```python
from build123d import *

# Parameters (mm, degrees)
F0_W      = 45.72
F0_H      = 7.62
F1_DEPTH  = 25.4
F2_DEPTH  = 25.4
F3_DEPTH  = 3.81
F4_R      = 5.08
F7_DEPTH  = 3.81
F10_DEPTH = 3.81
F11_R     = 1.27


with BuildPart() as f1:
    # F0 (on Front) → F1 (new body, symmetric)
    with BuildSketch(Plane.XZ):
        with Locations((-3.917041, 3.81)):
            Rectangle(F0_W, F0_H)
    extrude(amount=F1_DEPTH, both=True)

    # F0 (on Front) → F2 (join, symmetric)
    with BuildSketch(Plane.XZ):
        Polygon((26.562959, 38.1), (18.942959, 38.1), (18.942959, 7.62), (18.942959, 0), (18.942959, -7.62), (26.562959, -7.62), align=None)
    extrude(amount=F2_DEPTH, both=True)

    # F0 (on Front) → F3 (join, symmetric)
    with BuildSketch(Plane.XZ):
        with BuildLine():
            Line((18.942959, -7.62), (18.942959, 0))
            Line((18.942959, 0), (-26.777041, 0))
            add(Edge.make_bspline(
                [(-26.777041, 0), (-8.442144, -4.630308), (0.605608, -7.060291), (18.942959, -7.62)],
                knots=[0, 0, 0, 0, 46.35065, 46.35065, 46.35065, 46.35065], degree=3))
        make_face()
    extrude(amount=F3_DEPTH, both=True)

    # F4
    f4_edges = [f1.edges().sort_by_distance(p)[0] for p in [
        (22.752959, -25.4, -7.62),
        (22.752959, 25.4, -7.62),
        (22.752959, 25.4, 38.1),
        (22.752959, -25.4, 38.1),
        (-26.777041, 25.4, 3.81),
        (-26.777041, -25.4, 3.81),
    ]]
    fillet(f4_edges, radius=F4_R)

    # F6 (on offset) → F7 (join, symmetric)
    with BuildSketch(Plane.XZ.offset(12.7)):
        with BuildLine():
            Line((19.504473, 7.642324), (19.504473, 37.258741))
            add(Edge.make_bspline(
                [(19.504473, 37.258741), (-2.269479, 32.051925), (-15.974103, 23.058929), (-26.861079, 7.675159)],
                knots=[0, 0, 0, 0, 54.99957, 54.99957, 54.99957, 54.99957], degree=3))
            Line((-26.861079, 7.675159), (19.504473, 7.642324))
        make_face()
    extrude(amount=F7_DEPTH, both=True)

    # F9 (on offset) → F10 (join, symmetric)
    with BuildSketch(Plane.XZ.offset(-12.7)):
        with BuildLine():
            Line((19.418189, 7.557305), (19.418189, 37.171504))
            add(Edge.make_bspline(
                [(19.418189, 37.171504), (-2.355763, 31.964688), (-16.060385, 22.97391), (-26.947361, 7.590141)],
                knots=[0, 0, 0, 0, 54.998375, 54.998375, 54.998375, 54.998375], degree=3))
            Line((-26.947361, 7.590141), (19.418189, 7.557305))
        make_face()
    extrude(amount=F10_DEPTH, both=True)

    # F11
    f11_edges = [f1.edges().sort_by_distance(p)[0] for p in [
        (26.562959, 25.4, 15.24),
        (26.562959, 23.912102, -6.132102),
        (26.562959, 23.912102, 36.612102),
        (26.562959, 0, -7.62),
        (26.562959, 0, 38.1),
        (26.562959, -23.912102, -6.132102),
        (26.562959, -23.912102, 36.612102),
        (26.562959, -25.4, 15.24),
        (-6.865306, -16.51, 26.848425),
        (-6.865306, -8.89, 26.848425),
        (-6.913699, 16.51, 26.785701),
        (-6.913699, 8.89, 26.785701),
    ]]
    fillet(f11_edges, radius=F11_R)


solid = f1.part
```
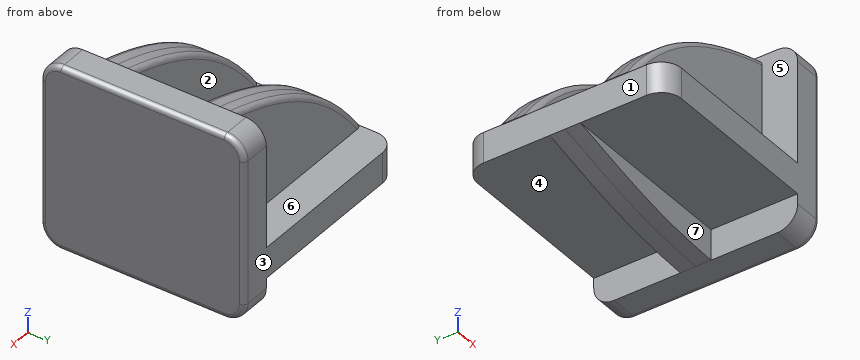
For this review, take the finished solid that the model builds, in its own axes (mm). Face numbers are marked on the shaded views. A direction names the side the tool comes from. Round coordinates to 2 decimals unless told otherwise and drop trailing zeros. Write each loop counter-clockwise with the first axis right and the second up, starting at its lowest first coordinate (ties: lowest second). Pieces come first, ordered by that corner, then holes. Notation, with made-up numbers: (70, -3.75) -> (84, -3.75) arc R19 cw to (84, 20.25) -> close; hole circle Ø3 at (0.5, 36.5). An arc over 180 degrees is marked (long way). One line per question, with ' | ' between items. Start each with the question number.
1) Add section A-A (y = -18). Write out the cut boundary in (x, z), and give its area (3 significant figures).
2) Wall thickness on line 1 along Y through (x, z) = (5.5, 23); line 2 along X through (y, z) = (-21, 26.5); line 3 along Z through (x, y) = (-24, -23): over which ranges is each line inside the solid? List them lowest first.
3) Machinability: for the marked faces 4, 5, 6 and 7, which of the approach directions +Z, -Z, +X, -X, +Y, -Y give a long, thin tool a straight path to every point of the face, cutting with its end or side? Answer none if there is none.
4) Mouldability with a two-part tool opening along Y and no side actions: class the marked faces 1, 2 and 3 as +Y half, -Y half, draft (parallel to the pull), parting line (faces both ways), or undercut.
5) For pin 1 Ø5 at (x, z) = (3.5, 24) entering from +Y; pin 2 Ø8.5 at (y, z) = (-18, -5) entering from -X; pin 3 Ø10 at (x, y) = (1.5, 7) entering from +Z, all flat-tipped, find the tip position at first contact; note any pin that passes through.
Reported:
1) outline: (-26.78, 0) -> (18.94, 0) -> (18.94, -7.62) -> (25.29, -7.62) arc R1.27 ccw to (26.56, -6.35) -> (26.56, 36.83) arc R1.27 ccw to (25.29, 38.1) -> (18.94, 38.1) -> (18.94, 7.62) -> (-26.78, 7.62) -> close | area: 696 mm²
2) line 1: y = -16.51 to -8.89, 8.89 to 16.51 | line 2: x = 18.94 to 26.56 | line 3: z = 0 to 7.62
3) face 4: -Z, -X, +Y | face 5: +Z, -X | face 6: +Z, -X, +Y | face 7: -Z, -X, -Y
4) face 1: draft | face 2: undercut | face 3: +Y half
5) pin 1: stops at y = 16.51 | pin 2: stops at x = 18.94 | pin 3: stops at z = 32.9
